Design review of the part built by this model. Coordinates are the model's own, in mm. A direction names the side the tool comes from. Coordinates: 2 decimals unless noted, no trailing zeros. Write each loop counter-clockwise with the first axis right and the second up, starting at its lowest first coordinate (ties: lowest second). Pieces come first, ordered by that corner, then holes.
Q1. Take a section at B-B (x = 69). Give the boundary of the cut face in (y, z), and give its area (3 significant figures).
Q2. For probe 1 along X at (y, z) = (104, 3.2); probe 2 along Y at (x, z) = (50, 1.5); probe 3 along Y at (x, z) = (89.5, 1.1), list the stretches that pass through material, from the lowest coordinate up.
Q3. Machinability: for faces 4 (the flat face through (200, 99, 2)), 5 (the flat face through (90, 75, 3)), which of the approach directions +Z, -Z, +X, -X, +Y, -Y give a long, thin tool a straight path to every point of the face, cutting with its end or side? Answer none if there is none.
Q4. Mouldability with a two-part tool opening along Y and no side actions: class faces 1 (the flat face through (11, 72.5, 3)), 2 (the flat face through (121, 101, 5)), 3 (the flat face through (99, 200, 2)) as pulls with the +Y half, pulls with the -Y half, needs draft (parallel to the pull), parting line crosses it, or undercut.
Q5. Take a section at A-A (z = 2.75). Give the boundary of the cut face in (x, y), and give its area (3 significant figures).
Q6. Insertion check: pin 1 (1.5 mm diameter, centred on x = 8.5, z = 3.5, fed in from -Y); pin 2 (3 mm diameter, centred on x = 130, y = 75, fed in from +Z). Each pin has a flat end and moves straight along its axis. Give the tip position at first contact, or say it passes through.
Q7. Take a section at C-C (y = 92). Give the boundary of the cut face in (x, z), and give its area (3 significant figures).
```python
from build123d import *

# Parameters (mm, degrees)
ESQUISSE1_W             = 200
ESQUISSE1_H             = 200
BOSS_EXTRU_1_DEPTH      = 5
ESQUISSE2_R             = 2
ENL_V_MAT_EXTRU_1_DEPTH = 10
ESQUISSE3_W             = 13
ESQUISSE3_H             = 55
ENL_V_MAT_EXTRU_2_DEPTH = 10
ESQUISSE4_W             = 60
ESQUISSE4_H             = 50
ENL_V_MAT_EXTRU_3_DEPTH = 12


with BuildPart() as part:
    # Esquisse1 → Boss.-Extru.1 (new body)
    with BuildSketch(Plane.XY):
        with Locations((100, 100)):
            Rectangle(ESQUISSE1_W, ESQUISSE1_H)
    extrude(amount=BOSS_EXTRU_1_DEPTH)

    # Esquisse2 → Enlèv. mat.-Extru.1 (cut)
    with BuildSketch(Plane.XY.offset(5)):
        with Locations((50, 125)):
            Circle(ESQUISSE2_R)
        with Locations((50, 75)):
            Circle(ESQUISSE2_R)
        with Locations((130, 125)):
            Circle(ESQUISSE2_R)
        with Locations((130, 75)):
            Circle(ESQUISSE2_R)
    extrude(amount=-ENL_V_MAT_EXTRU_1_DEPTH, mode=Mode.SUBTRACT)

    # Esquisse3 → Enlèv. mat.-Extru.2 (cut)
    with BuildSketch(Plane.XY.offset(5)):
        with Locations((11.5, 100)):
            Rectangle(ESQUISSE3_W, ESQUISSE3_H)
    extrude(amount=-ENL_V_MAT_EXTRU_2_DEPTH, mode=Mode.SUBTRACT)

    # Esquisse4 → Enlèv. mat.-Extru.3 (cut)
    with BuildSketch(Plane.XY.offset(5)):
        with Locations((90, 100)):
            Rectangle(ESQUISSE4_W, ESQUISSE4_H)
    extrude(amount=-ENL_V_MAT_EXTRU_3_DEPTH, mode=Mode.SUBTRACT)


solid = part.part
```
Response:
1. outline: (0, 0) - (75, 0) - (75, 5) - (0, 5) - close; (125, 0) - (200, 0) - (200, 5) - (125, 5) - close
1. area: 750 mm2
2. probe 1: x = 0 to 5, 18 to 60, 120 to 200
2. probe 2: y = 0 to 73, 77 to 123, 127 to 200
2. probe 3: y = 0 to 75, 125 to 200
3. face 4: +Z, -Z, +X, +Y, -Y
3. face 5: +Z, -Z
4. face 1: undercut
4. face 2: needs draft
4. face 3: pulls with the +Y half
5. outline: (0, 0) - (200, 0) - (200, 200) - (0, 200) - close; hole (5, 72.5) - (18, 72.5) - (18, 127.5) - (5, 127.5) - close; hole circle Ø4 at (50, 75); hole circle Ø4 at (50, 125); hole (60, 75) - (120, 75) - (120, 125) - (60, 125) - close; hole circle Ø4 at (130, 75); hole circle Ø4 at (130, 125)
5. area: 36,200 mm2
6. pin 1: stops at y = 0
6. pin 2: passes through
7. outline: (0, 0) - (5, 0) - (5, 5) - (0, 5) - close; (18, 0) - (60, 0) - (60, 5) - (18, 5) - close; (120, 0) - (200, 0) - (200, 5) - (120, 5) - close
7. area: 635 mm2
